The drawing under review shows one solid part. Ordinate dimensions are in mm from its lowest x, y, z. A direction names the side the tool comes from. Round coordinates to 2 decimals unless told otherwise and drop trailing zeros. Order: outer loops, then holes, each group sorted by start corner. A loop starts at its lowest first (then second) coordinate and runs counter-clockwise, first axis right, second up. Notation, with made-up numbers: M 63.5,21.5 L 115.5,21.5 A19 cw 115.5,29.5 Z; hole C -19.75,67.25 d10. An arc over 180 degrees is marked long. Answer as a JSON object with one key per item and string values.
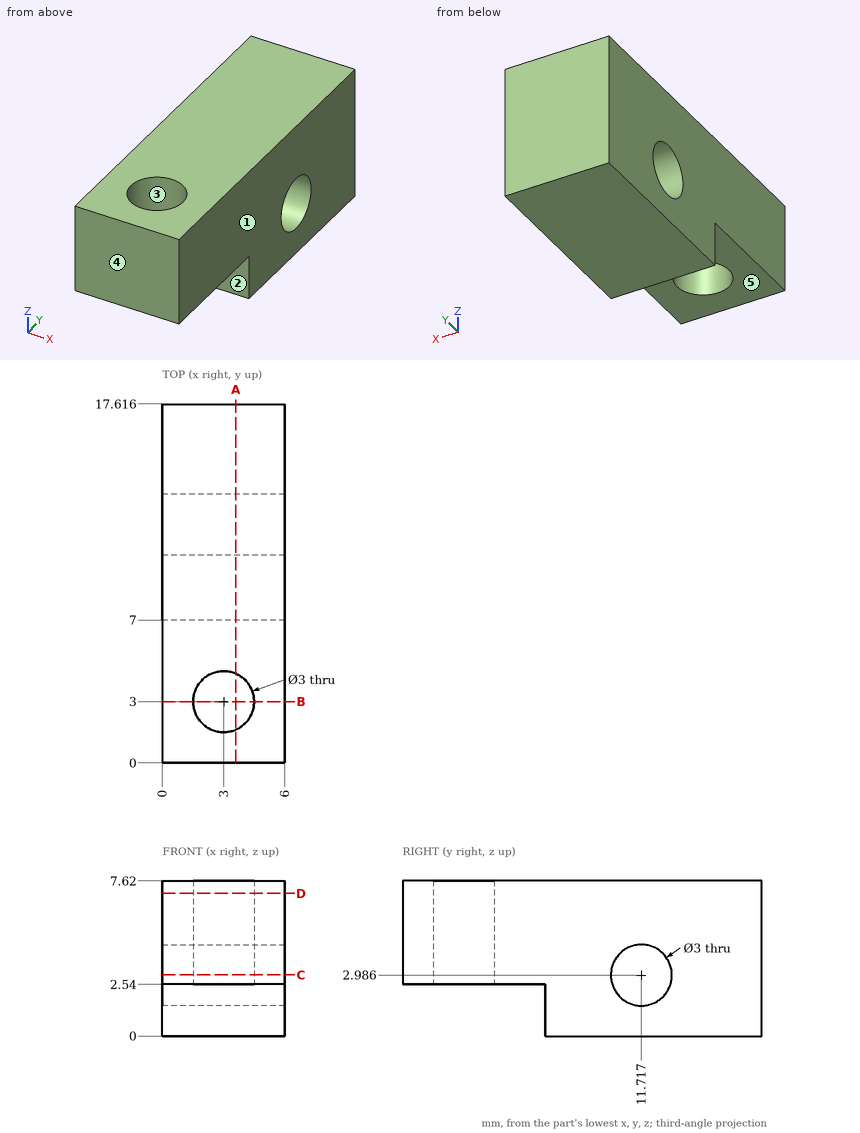
1) Add section A-A on x = 3.6. State the section outline as (y, z) points (1 decimal).
Geometry check:
{"outline": "M 0,2.5 L 1.6,2.5 L 1.6,7.6 L 0,7.6 Z; M 4.4,2.5 L 7,2.5 L 7,0 L 17.6,0 L 17.6,7.6 L 4.4,7.6 Z; hole C 11.7,3 d3"}
2) Machinability: for the marked faces 4 and 5, which of the approach directions +Z, -Z, +X, -X, +Y, -Y give a long, thin tool a straight path to every point of the face, cutting with its end or side? Answer none if there is none.
Geometry check:
{"face 4": "+Z, -Z, +X, -X, -Y", "face 5": "-Z, +X, -X, -Y"}
3) Insertion check: P1, Ø1.8, axis at x = 3.5, y = 2, coming from the -Z side; P2, Ø0.8, axis at x = 2.5, z = 0.5, coming from the -Y side. Each pin has a flat end and moves straight along its axis. Give the tip position at first contact, or say it passes through.
Geometry check:
{"P1": "stops at z = 2.54", "P2": "stops at y = 7"}
4) Add section C-C on z = 3. State the section outline as (x, y) points (1 decimal).
Geometry check:
{"outline": "M 0,0 L 6,0 L 6,10.2 L 0,10.2 Z; M 0,13.2 L 6,13.2 L 6,17.6 L 0,17.6 Z; hole C 3,3 d3"}
5) Mouldability with a two-part tool opening along X and no side actions: class the marked faces 1, 2 and 3 as +X half, -X half, draft (parallel to the pull), parting line (faces both ways), or undercut.
Geometry check:
{"face 1": "+X half", "face 2": "draft", "face 3": "undercut"}
6) For L1, parallel to X at y = 3, z = 5.5; L2, parallel to Y at x = 0.7, z = 3 (1 decimal); L3, parallel to Y at x = 3, z = 3.7 (1 decimal), list the stretches that pass through material, from the lowest coordinate up.
Geometry check:
{"L1": "x = 0 to 1.5, 4.5 to 6", "L2": "y = 0 to 10.2, 13.2 to 17.6", "L3": "y = 0 to 1.5, 4.5 to 10.4, 13 to 17.6"}
7) Add section D-D on z = 7. State the section outline as (x, y) points (1 decimal).
Geometry check:
{"outline": "M 0,0 L 6,0 L 6,17.6 L 0,17.6 Z; hole C 3,3 d3"}
8) Add section B-B on y = 3. State the section outline as (x, z) points.
Geometry check:
{"outline": "M 0,2.54 L 1.5,2.54 L 1.5,7.62 L 0,7.62 Z; M 4.5,2.54 L 6,2.54 L 6,7.62 L 4.5,7.62 Z"}
